```python
from build123d import *

# Parameters (mm, degrees)
SKETCH1_W           = 50
SKETCH1_H           = 50
BOSS_EXTRUDE1_DEPTH = 52.13
CUT_EXTRUDE1_DEPTH  = 52.13
SKETCH3_W           = 50
SKETCH3_H           = 38
CUT_EXTRUDE2_DEPTH  = 52.13
BOSS_EXTRUDE3_DEPTH = 38
SKETCH5_R           = 11
CUT_EXTRUDE3_DEPTH  = 52.13


with BuildPart() as part:
    # Sketch1 → Boss-Extrude1 (new body)
    with BuildSketch(Plane(origin=(0, 0, 0), x_dir=(1, 0, 0), z_dir=(0, 1, 0))):
        with Locations((25, 25)):
            Rectangle(SKETCH1_W, SKETCH1_H)
    extrude(amount=BOSS_EXTRUDE1_DEPTH)

    # Sketch2 → Cut-Extrude1 (cut)
    with BuildSketch(Plane.XY):
        Polygon((0, 32.13), (0, 0), (38.31009136, 0), align=None)
    extrude(amount=-CUT_EXTRUDE1_DEPTH, mode=Mode.SUBTRACT)

    # Sketch3 → Cut-Extrude2 (cut)
    with BuildSketch(Plane(origin=(0, 52.13, 0), x_dir=(1, 0, 0), z_dir=(0, 1, 0))):
        with Locations((25, 25)):
            Rectangle(SKETCH3_W, SKETCH3_H)
    extrude(amount=-CUT_EXTRUDE2_DEPTH, mode=Mode.SUBTRACT)

    # Sketch4 → Boss-Extrude3 (add)
    with BuildSketch(Plane.XY.offset(-44)):
        Polygon((6, 34.928740389), (6, 52.13), (0, 52.13), (0, 32.13), (38.31009136, 0), (50, 0), (50, 6), (40.493080835, 6), align=None)
    extrude(amount=BOSS_EXTRUDE3_DEPTH)

    # Sketch5 → Cut-Extrude3 (cut)
    with BuildSketch(Plane(origin=(15.819568381, 18.862406161, 0), x_dir=(0.766201827, -0.6426, 0), z_dir=(-0.6426, -0.766201827, 0))):
        with Locations((4.353262, -25)):
            Circle(SKETCH5_R)
    extrude(amount=-CUT_EXTRUDE3_DEPTH, mode=Mode.SUBTRACT)


solid = part.part
```
Geometry: final body of the model. Coordinates: model frame, mm. A direction names the side the tool comes from. Coordinates: 2 decimals unless noted, no trailing zeros. Loops run counter-clockwise (first coordinate to the right, second up) from the corner with the lowest first, then second, coordinate; pieces in that order, holes last. Notation, with made-up numbers: M 55,27 L 79,27 A13 cw 79,47 Z; hole C 17.25,31 d8. An arc over 180 degrees is marked long. Put each result on its own line as item: value.
(1) Draft query along Z for faces 1 (the face through (45, 6, -25)), 2 (the face through (44, 0, -25)), 3 (the face through (30, 31, -50)). Return one class per face: pulls with the +Z half, pulls with the -Z half, needs draft (parallel to the pull), parting line crosses it, or undercut.
Answer sheet:
face 1: undercut
face 2: needs draft
face 3: pulls with the -Z half
(2) Cut plane C-C on y = 7. Return the cut outline in (x, z), then the cut area to 3 significant figures.
Answer sheet:
outline: M 29.96,-50 L 50,-50 L 50,-44 L 39.3,-44 L 39.3,-6 L 50,-6 L 50,0 L 29.96,0 Z
area: 595 mm^2
(3) Cut plane B-B on x = 42. Return the cut outline in (y, z), then the cut area to 3 significant figures.
Answer sheet:
outline: M 0,-50 L 52.13,-50 L 52.13,-44 L 6,-44 L 6,-6 L 52.13,-6 L 52.13,0 L 0,0 Z
area: 854 mm^2
(4) Access query for faces 4 (the face through (18.887, 16.29, -36.461)), 5 (the face through (6, 43, -25)). Directions: +Z, -Z, +X, -X, +Y, -Y. A direction counts if a zero-diameter tool reaches every point of the face in a straight line with its end or side. Return the directions, or none.
Answer sheet:
face 4: +Z, -Z, -X, -Y
face 5: +X, +Y
(5) Material intervals for probe 1 along Z at (x, y) = (18, 48.5); probe 2 along X at (y, z) = (42.5, -27), sorted ascending.
Answer sheet:
probe 1: z = -50 to -44, -6 to 0
probe 2: x = 0 to 6
(6) Cut plane A-A on z = -32. Return the cut outline in (x, y), then the cut area to 3 significant figures.
Answer sheet:
outline: M 0,32.13 L 12.65,21.52 L 16.51,26.11 L 6,34.93 L 6,52.13 L 0,52.13 Z; M 25.66,10.61 L 38.31,0 L 50,0 L 50,6 L 40.49,6 L 29.51,15.21 Z
area: 358 mm^2
(7) First-contact query: pin 1 (1.5 mm diameter, centred on y = 41, z = -8, fed in from +X); pin 2 (1.5 mm diameter, centred on x = 16, z = -36.5, fed in from +Y); pin 3 (10.5 mm diameter, centred on x = 45, z = -30, fed in from +Y). Flat tips, straight axial feed; report the tip coordinate or a pass-through.
Answer sheet:
pin 1: stops at x = 6
pin 2: stops at y = 27.17
pin 3: stops at y = 6.62
